Here's how the part is built. I have some questions about the finished solid (model axes, mm). Round coordinates to 2 decimals unless told otherwise and drop trailing zeros. Write each loop counter-clockwise with the first axis right and the second up, starting at its lowest first coordinate (ties: lowest second). Pieces come first, ordered by that corner, then holes. Notation, with made-up numbers: (-20, 35.25) - (-9, 35.25) arc R5 ccw to (-9, 43.25) - close; hole circle Ø6 at (-3, 72.25). An arc over 180 degrees is marked (long way). Write item = value, one per line. Start each with the question number.
Item 1: If we section it at B-B (y = 0): Please give me the cut outline in (x, z), and give its area (3 significant figures).
Item 2: If we section it at A-A (x = 0): Please give me the cut outline in (y, z) (3 decimals).
Item 3: If we section it at C-C (z = 3.25): Please give me the cut outline in (x, y), and give its area (3 significant figures).
Item 4: If I drill on line 1 along Z through (x, y) = (0, 9.25) (3 decimals); line 2 along Y through (x, z) = (0, 8.5); line 3 along X through (y, z) = (11.5, 5.55) (3 decimals), over which ranges is the centre line in solid material (lowest first)? Write a range as [from, to].
Item 5: If we section it at D-D (z = 6.5): Please give me the cut outline in (x, y).
Item 6: Thinking about a two-plate mould opening in X: for faces 1 (the face through (2.822, 9.144, 5.426)), 2 (the face through (5, -5, 0)), 3 (the face through (6.827, -10.709, 5.486)), which applies, pulls with the +X half, pulls with the -X half, needs draft (parallel to the pull), parting line crosses it, or undercut?
Item 7: For P1, Ø5, axis at y = -8, z = 4, coming from the -X side; P2, Ø3.5, axis at x = 0, z = 5.55, coming from the +Y side; P3, Ø1, axis at y = 2, z = 8, coming from the -X side, each with a flat end and sliding along its axis, tell me the tip position at first contact or that it passes through.
Autodesk Inventor part; units mm, degrees
ref_plane "YZ Plane" through (0, 0, 0) normal (1, 0, 0) x (0, 1, 0)
ref_plane "XZ Plane" through (0, 0, 0) normal (0, 1, 0) x (-1, 0, 0)
ref_plane "XY Plane" through (0, 0, 0) normal (0, 0, 1) x (1, 0, 0)
sketch "Sketch1" plane through (0, 0, 0) normal (0, 0, 1) x (1, 0, 0)
  circle A0 centre (0, 0) radius 12.7
  circle A1 centre (0, 0) radius 6.35
  dimension "d0" = 25.4
  dimension "d1" = 12.7
extrude "Extrusion1" add sketch "Sketch1" along normal blind 11.1
sketch "Sketch2" plane through (0, 0, 0) normal (0, 1, 0) x (-1, 0, 0)
  circle A0 centre (0, 5.55) radius 2.825
  line L0 (12.7, 0) -> (12.7, 11.1)
  point P0 (0, 0)
  point P1 (12.7, 5.55)
  dimension "d4" = 5.65
extrude "Extrusion2" cut sketch "Sketch2" along normal through all
fillet "Fillet1" radius 1 2 edges at (-12.7, 0, 11.1) (-12.7, 0, 0)
thread "Thread1"
properties part number "Shaft Collar" material "ABS Plastic"
Reply:
q1.outline = (-12.7, 1) arc R1 ccw to (-11.7, 0) - (-6.35, 0) - (-6.35, 11.1) - (-11.7, 11.1) arc R1 ccw to (-12.7, 10.1) - close; (6.35, 0) - (11.7, 0) arc R1 ccw to (12.7, 1) - (12.7, 10.1) arc R1 ccw to (11.7, 11.1) - (6.35, 11.1) - close
q1.area = 140 mm2
q2.outline = (-12.7, 1) arc R1 ccw to (-11.7, 0) - (-6.35, 0) - (-6.35, 11.1) - (-11.7, 11.1) arc R1 ccw to (-12.7, 10.1) - close; (6.35, 0) - (11.7, 0) arc R1 ccw to (12.7, 1) - (12.7, 2.725) - (6.35, 2.725) - close; (6.35, 8.375) - (12.7, 8.375) - (12.7, 10.1) arc R1 ccw to (11.7, 11.1) - (6.35, 11.1) - close
q3.outline = (-1.64, 6.13) - (-1.64, 12.59) arc R12.7 ccw (long way) to (1.64, 12.59) - (1.64, 6.13) arc R6.35 cw (long way) to start
q3.area = 359 mm2
q4.line_1 = [0, 2.725], [8.375, 11.1]
q4.line_2 = [-12.7, -6.35], [6.35, 12.7]
q4.line_3 = [-5.389, -2.825], [2.825, 5.389]
q5.outline = (-2.66, 5.77) - (-2.66, 12.42) arc R12.7 ccw (long way) to (2.66, 12.42) - (2.66, 5.77) arc R6.35 cw (long way) to start
q6.face_1 = undercut
q6.face_2 = needs draft
q6.face_3 = parting line crosses it
q7.P1 = -11.45
q7.P2 = -6.1
q7.P3 = -12.61
